Verification items for this drawing (mm, ordinates from the low corner). A direction names the side the tool comes from. Round coordinates to 2 decimals unless told otherwise and drop trailing zeros. Order: outer loops, then holes, each group sorted by start corner. A loop starts at its lowest first (then second) coordinate and runs counter-clockwise, first axis right, second up. Notation, with made-up numbers: (32.5, 87) -> (48.5, 87) arc R13 cw to (48.5, 94) -> close; hole circle Ø2 at (32, 3.25). An arc over 180 degrees is marked (long way). Use a Markdown table: item, result. Add a question column.
Item 1: Sectioned sample at C-C, the plane x = 10. Record the cut outline in (y, z), and give its area (3 significant figures).
Item 2: Gauge pin test, flat ends, axial feed: pin 1 Ø3 at (x, z) = (10.5, 62.5) entering from -Y; pin 2 Ø2 at (x, z) = (21, 24) entering from +Y; pin 3 Ø2 at (x, z) = (13, 61.5) entering from +Y; pin 4 Ø8 at (x, z) = (11, 46) entering from -Y. Record the tip position at first contact, or that the pin passes through.
Item 3: Sectioned sample at A-A, the plane y = 49.5. Record the cut outline in (x, z).
Item 4: Set-up check for the marked faces 4 and 5: record each of +Z, -Z, +X, -X, +Y, -Y from which the full face is reachable in a straight line by a thin tool's end or side.
Item 5: Mould release check, pull along Z, two halves, no side actions. Record for the marked faces 1, 2 and 3: pulls with the +Z half, pulls with the -Z half, needs draft (parallel to the pull), parting line crosses it, or undercut.
Item 6: Material ranges on probe 1 along Z at (x, y) = (23.3, 49.5); probe 2 along Z at (x, y) = (2.1, 49.5); probe 3 along X at (y, z) = (59, 75), recorded low to high. Write a range as [from, to].
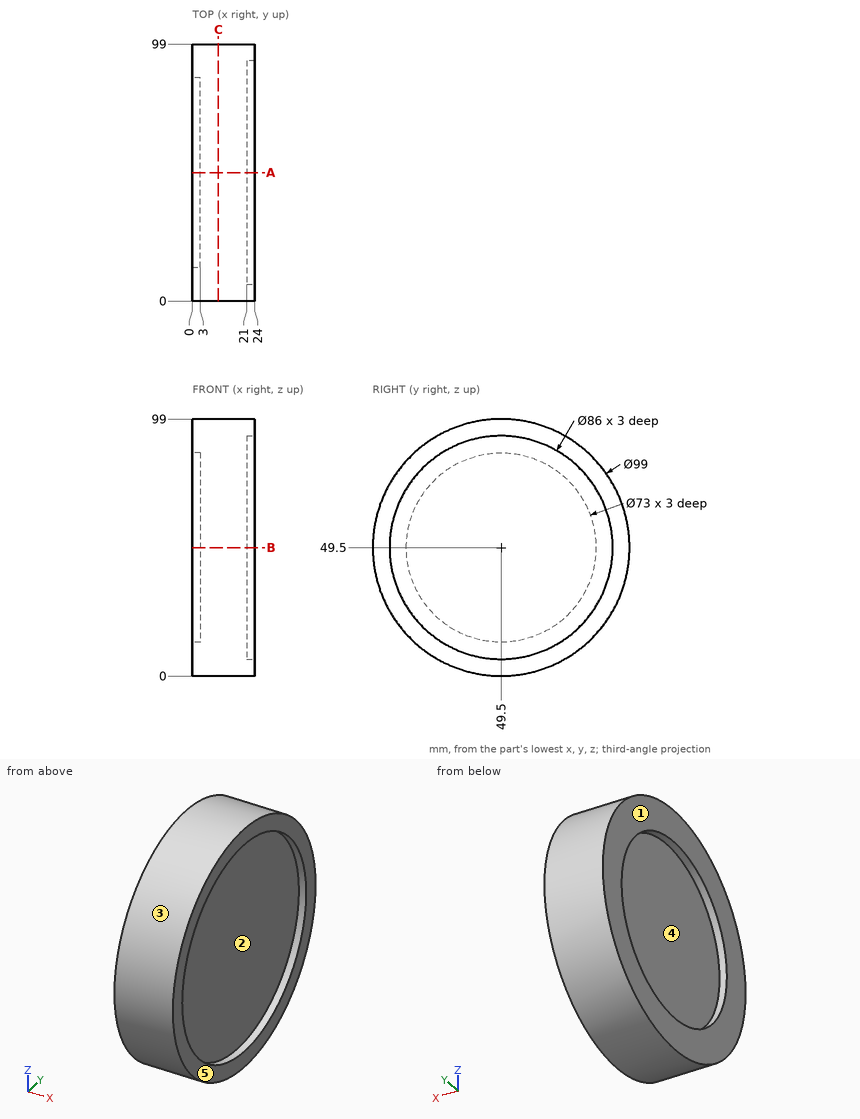
Found:
| question | item | result |
|---|---|---|
| 1 | outline | circle Ø99 at (49.5, 49.5) |
| 1 | area | 7,700 mm2 |
| 2 | pin 1 | stops at y = 1.35 |
| 2 | pin 2 | stops at y = 92.51 |
| 2 | pin 3 | stops at y = 97.76 |
| 2 | pin 4 | stops at y = 0 |
| 3 | outline | (0, 0) -> (24, 0) -> (24, 6.5) -> (21, 6.5) -> (21, 92.5) -> (24, 92.5) -> (24, 99) -> (0, 99) -> (0, 86) -> (3, 86) -> (3, 13) -> (0, 13) -> close |
| 4 | face 4 | -X |
| 4 | face 5 | +Z, -Z, +X, +Y, -Y |
| 5 | face 1 | needs draft |
| 5 | face 2 | undercut |
| 5 | face 3 | parting line crosses it |
| 6 | probe 1 | z = [0, 6.5], [92.5, 99] |
| 6 | probe 2 | z = [0, 13], [86, 99] |
| 6 | probe 3 | x = [3, 21] |
